```python
from build123d import *

# Parameters (mm, degrees)
SKETCH1_W           = 54
SKETCH1_H           = 25
SKETCH1_R           = 1.75
BOSS_EXTRUDE1_DEPTH = 2
SKETCH2_W           = 54
SKETCH2_H           = 2.5
BOSS_EXTRUDE2_DEPTH = 27
SKETCH3_W           = 54
SKETCH3_H           = 2.5
BOSS_EXTRUDE3_DEPTH = 2
SKETCH4_R           = 1.75
CUT_EXTRUDE1_DEPTH  = 27
FILLET1_R           = 5


with BuildPart() as part:
    # Sketch1 → Boss-Extrude1 (new body)
    with BuildSketch(Plane(origin=(0, 0, 0), x_dir=(1, 0, 0), z_dir=(0, 1, 0))):
        with Locations((27, 12.5)):
            Rectangle(SKETCH1_W, SKETCH1_H)
        with Locations(Location((4, 4, 0), (0, 0, 270))):
            Circle(SKETCH1_R, mode=Mode.SUBTRACT)
        with Locations(Location((50, 4, 0), (0, 0, 270))):
            Circle(SKETCH1_R, mode=Mode.SUBTRACT)
    extrude(amount=BOSS_EXTRUDE1_DEPTH)



with BuildPart() as body_2:
    # Sketch2 → Boss-Extrude2 (new body)
    with BuildSketch(Plane(origin=(0, 2, 0), x_dir=(1, 0, 0), z_dir=(0, 1, 0))):
        with Locations((27, 26.25)):
            Rectangle(SKETCH2_W, SKETCH2_H)
    extrude(amount=BOSS_EXTRUDE2_DEPTH)


with BuildPart() as part_1:
    add(part.part)

    add(body_2.part)  # Boss-Extrude3 merges body 2
    # Sketch3 → Boss-Extrude3 (add)
    with BuildSketch(Plane.XZ.offset(-2)):
        with Locations((27, -26.25)):
            Rectangle(SKETCH3_W, SKETCH3_H)
    extrude(amount=BOSS_EXTRUDE3_DEPTH)

    # Sketch4 → Cut-Extrude1 (cut)
    with BuildSketch(Plane.XY.offset(-25)):
        with Locations((5.25, 19)):
            Circle(SKETCH4_R)
        with Locations((48.75, 19)):
            Circle(SKETCH4_R)
    extrude(amount=-CUT_EXTRUDE1_DEPTH, mode=Mode.SUBTRACT)

    # Fillet1
    fillet1_edges = [part_1.edges().sort_by_distance(p)[0] for p in [
        (27, 2, -25),
    ]]
    fillet(fillet1_edges, radius=FILLET1_R)


solid = part_1.part
```
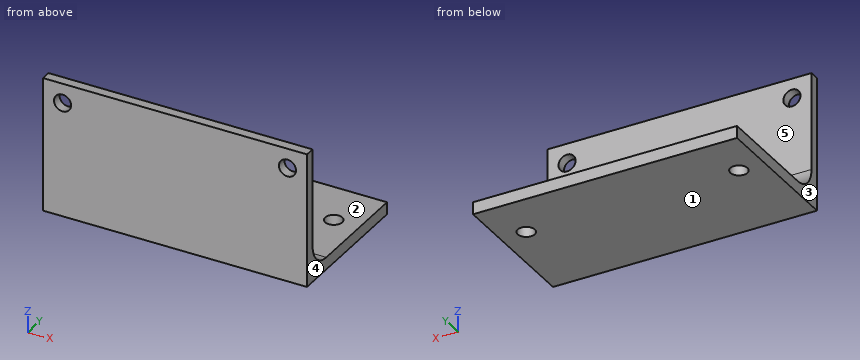
Check sheet for the modelled part. Datum: model origin and axes. Units: mm. Face numbers are marked on the shaded views. A direction names the side the tool comes from. Give positions to 0.01 mm unless a question says otherwise; leave off trailing zeros. Order: outer loops, then holes, each group sorted by start corner. A loop starts at its lowest first (then second) coordinate and runs counter-clockwise, first axis right, second up. Notation, with made-up numbers: (12.25, 82.5) -> (58.25, 82.5) arc R23 cw to (58.25, 112.5) -> close; hole circle Ø4 at (-25, 24.25). An arc over 180 degrees is marked (long way). Return JSON: item names as keys, results as strings.
1. Cross-section at B-B, the plane y = 19. Record the cut outline in (x, z), plus the area to 4 significant figures.
From the geometry:
{"outline": "(0, -27.5) -> (3.5, -27.5) -> (3.5, -25) -> (0, -25) -> close; (7, -27.5) -> (47, -27.5) -> (47, -25) -> (7, -25) -> close; (50.5, -27.5) -> (54, -27.5) -> (54, -25) -> (50.5, -25) -> close", "area": "117.5 mm^2"}
2. Mould release check, pull along Z, two halves, no side actions. Record for the marked faces 1, 2 and 3: +Z half, -Z half, draft (parallel to the pull), parting line (faces both ways), or undercut.
From the geometry:
{"face 1": "-Z half", "face 2": "+Z half", "face 3": "draft"}
3. Go/stop test with flat-tipped pins: P1, Ø4, axis at y = 24, z = -23.5, coming from the +X side; P2, Ø2, axis at x = 23, z = -4, coming from the +Y side; P3, Ø8, axis at x = 15.5, y = 9, coming from the +Z side; P4, Ø5, axis at x = 46, y = 7, coming from the +Z side. Record where each tip stops, or that it passes through.
From the geometry:
{"P1": "x = 54", "P2": "y = 2", "P3": "z = -24.58", "P4": "z = -24.33"}
4. Cross-section at D-D, the plane z = -16.5. Record the cut outline in (x, y).
From the geometry:
{"outline": "(0, 0) -> (54, 0) -> (54, 2) -> (0, 2) -> close"}
5. Cross-section at A-A, the plane z = -4. Record the cut outline in (x, y), plus the area to 3 significant figures.
From the geometry:
{"outline": "(0, 0) -> (2.25, 0) -> (2.25, 2) -> (0, 2) -> close; (5.75, 0) -> (48.25, 0) -> (48.25, 2) -> (5.75, 2) -> close; (51.75, 0) -> (54, 0) -> (54, 2) -> (51.75, 2) -> close", "area": "94.0 mm^2"}
6. Cross-section at C-C, the plane x = 30. Record the cut outline in (y, z), plus the area to 3 significant figures.
From the geometry:
{"outline": "(0, -27.5) -> (29, -27.5) -> (29, -25) -> (7, -25) arc R5 cw to (2, -20) -> (2, 0) -> (0, 0) -> close", "area": "128 mm^2"}
7. Material ranges on probe 1 along Y at (x, z) = (5.25, -26.8); probe 2 along Y at (x, z) = (44.5, -5); probe 3 along Z at (x, y) = (46, 8), recorded low to high. Write a range as [from, to].
From the geometry:
{"probe 1": "[0, 17.25], [20.75, 29]", "probe 2": "[0, 2]", "probe 3": "[-27.5, -25]"}
8. Set-up check for the marked faces 4 and 5: record each of +Z, -Z, +X, -X, +Y, -Y from which the full face is reachable in a straight line by a thin tool's end or side.
From the geometry:
{"face 4": "+Z, -Z, +X, +Y, -Y", "face 5": "+Z, +X, -X, +Y"}
